Model file for the job. Use its own axes, mm. A direction names the side the tool comes from. Give positions to 0.01 mm unless a question says otherwise; leave off trailing zeros. Loops run counter-clockwise (first coordinate to the right, second up) from the corner with the lowest first, then second, coordinate; pieces in that order, holes last. Notation, with made-up numbers: (76, 49) - (81, 49) arc R20 ccw to (81, 78) - close; hole circle Ø6 at (36.5, -30.5). An arc over 180 degrees is marked (long way). Answer as CSV lines item,"result". Start each with the question number.
Item 1: Drill centre lines: L1, parallel to Z at x = 19.5, y = 3.5 (3 decimals); L2, parallel to Z at x = 13, y = 6; L3, parallel to X at y = 3.5, z = -23. Where is each one in solid material? Low to high. Write a range as from..to.
Item 2: Saw through at B-B on y = 4.75. Give the cut face in (x, z) (3 decimals), plus the area to 3 significant figures.
Item 3: Tool access for faces 4 (the flat face through (25, 3, -9.525)), 5 (the flat face through (2.88, 3.131, -25.105)), 6 (the flat face through (0, 0, -16)): list every direction of +Z, -Z, +X, -X, +Y, -Y with a clear straight run to the whole face (end or side of a thin tool).
Item 4: Saw through at D-D on z = -10.5. Give the cut face in (x, y), plus the area to 3 significant figures.
Item 5: Saw through at C-C on x = 20. Give the cut face in (y, z) (3 decimals), plus the area to 3 significant figures.
Item 6: Pull direction Z, two halves, no side cores. Call faces 1 (the flat face through (28.6, 3.1, -3.2)), 2 (the flat face through (31.75, 3, -24)), 3 (the flat face through (1.27, 3, -16)): pulls with the +Z half, pulls with the -Z half, needs draft (parallel to the pull), parting line crosses it, or undercut.
Item 7: Pin check, flat tip, straight feed: pin 1 (1.9 mm diameter, centred on y = 3, z = -15.5, fed in from +X). Stop position of the tip, or through.
Item 8: Saw through at A-A on x = 26.5. Give the cut face in (y, z) (3 decimals), plus the area to 3 significant figures.
Autodesk Inventor part; units mm, degrees
ref_plane "YZ Plane" through (0, 0, 0) normal (1, 0, 0) x (0, 1, 0)
ref_plane "XZ Plane" through (0, 0, 0) normal (0, 1, 0) x (-1, 0, 0)
ref_plane "XY Plane" through (0, 0, 0) normal (0, 0, 1) x (1, 0, 0)
sketch "Sketch1" plane through (0, 0, 0) normal (0, 1, 0) x (-1, 0, 0)
  line L0 (0, 0) -> (6.35, -6.35)
  line L1 (6.35, -6.35) -> (6.35, -25.4)
  line L2 (6.35, -25.4) -> (0, -31.75)
  line L3 (0, -31.75) -> (-25.4, -31.75)
  line L4 (-25.4, -31.75) -> (-31.75, -25.4)
  line L5 (-31.75, -25.4) -> (-31.75, -22.225)
  line L6 (-31.75, -22.225) -> (-19.05, -22.225)
  line L7 (-19.05, -22.225) -> (-19.05, -26.67)
  line L8 (-19.05, -26.67) -> (-4.445, -26.67)
  line L9 (-4.445, -26.67) -> (-1.27, -23.495)
  line L10 (-1.27, -23.495) -> (-1.27, -8.255)
  line L11 (-1.27, -8.255) -> (-4.445, -5.08)
  line L12 (-4.445, -5.08) -> (-19.05, -5.08)
  line L13 (-19.05, -5.08) -> (-19.05, -9.525)
  line L14 (-19.05, -9.525) -> (-31.75, -9.525)
  line L15 (-31.75, -9.525) -> (-31.75, -6.35)
  line L16 (-31.75, -6.35) -> (-25.4, 0)
  line L17 (-25.4, 0) -> (0, 0)
  dimension "d0" = 45
  dimension "d1" = 38.1
  dimension "d2" = 31.75
  dimension "d3" = 9.525
  dimension "d4" = 5.08
  dimension "d5" = 12.7
  dimension "d6" = 5.08
  dimension "d7" = 3.175
  dimension "d8" = 7.62
  dimension "d9" = 6.35
  dimension "d10" = 31.75
  dimension "d11" = 12.7
extrude "Extrusion1" add sketch "Sketch1" along normal blind 6.35
properties part number "C-Clip"
Responses:
1,L1,"-31.75..-22.225, -9.525..0"
1,L2,"-31.75..-26.67, -5.08..0"
1,L3,"-6.35..1.27, 19.05..31.75"
2,outline,"(-6.35, -25.4) - (0, -31.75) - (25.4, -31.75) - (31.75, -25.4) - (31.75, -22.225) - (19.05, -22.225) - (19.05, -26.67) - (4.445, -26.67) - (1.27, -23.495) - (1.27, -8.255) - (4.445, -5.08) - (19.05, -5.08) - (19.05, -9.525) - (31.75, -9.525) - (31.75, -6.35) - (25.4, 0) - (0, 0) - (-6.35, -6.35) - close"
2,area,"594 mm2"
3,face 4,"+X, +Y, -Y"
3,face 5,"+Y, -Y"
3,face 6,"+Z, -Z, +X, -X, -Y"
4,outline,"(-6.35, 0) - (1.27, 0) - (1.27, 6.35) - (-6.35, 6.35) - close"
4,area,"48.4 mm2"
5,outline,"(0, -31.75) - (6.35, -31.75) - (6.35, -22.225) - (0, -22.225) - close; (0, -9.525) - (6.35, -9.525) - (6.35, 0) - (0, 0) - close"
5,area,"121 mm2"
6,face 1,"pulls with the +Z half"
6,face 2,"needs draft"
6,face 3,"undercut"
7,pin 1,"x = 1.27"
8,outline,"(0, -30.65) - (6.35, -30.65) - (6.35, -22.225) - (0, -22.225) - close; (0, -9.525) - (6.35, -9.525) - (6.35, -1.1) - (0, -1.1) - close"
8,area,"107 mm2"
